The drawing under review shows one solid part. Ordinate dimensions are in mm from its lowest x, y, z. Give positions to 0.01 mm unless a question says otherwise; leave off trailing zeros. Order: outer loops, then holes, each group sorted by start corner. A loop starts at its lowest first (then second) coordinate and runs counter-clockwise, first axis right, second up. Notation, with made-up numbers: (18.25, 25.25) -> (51.25, 25.25) arc R12 cw to (51.25, 42.25) -> close; hole circle Ø5 at (29, 30.5). An arc over 180 degrees is marked (long way). One line per item, written item: value.
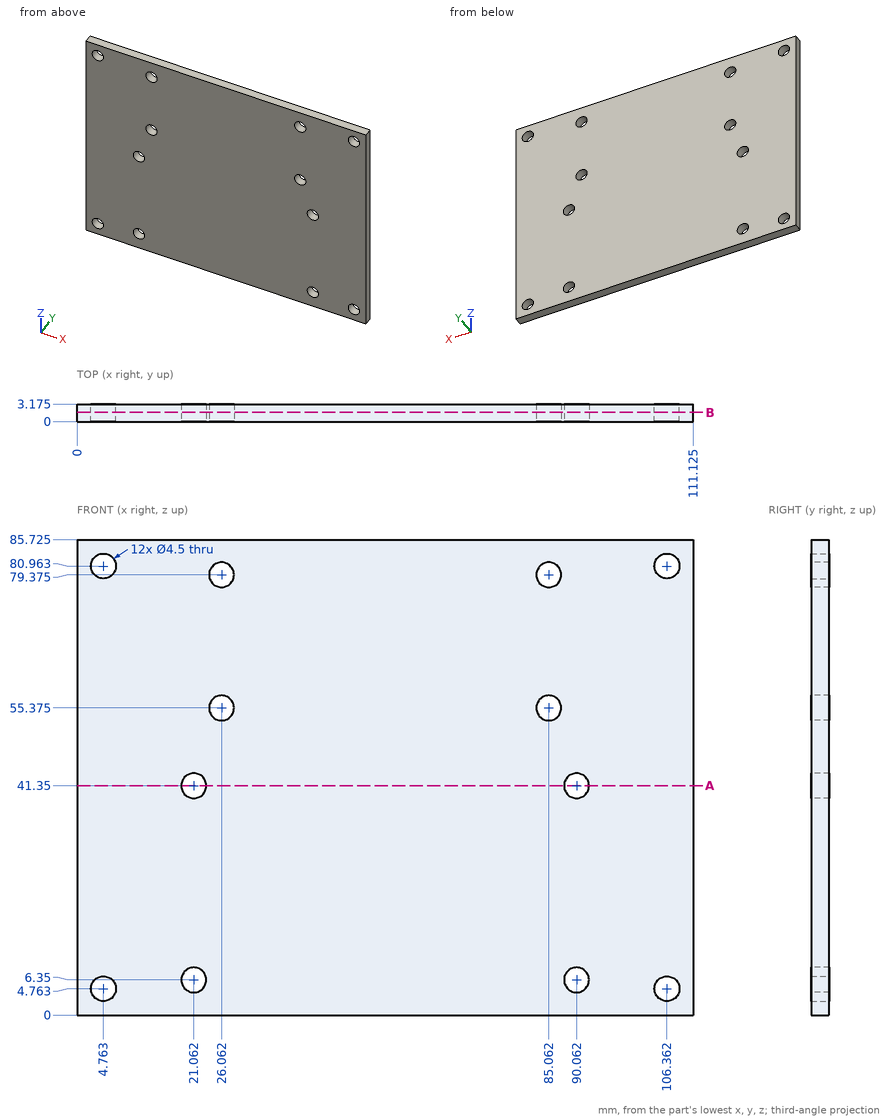
Item 1: Add section A-A on z = 41.35. Give the boundary of the cut face in (x, y) (1 decimal), plus the area to 3 significant figures.
Returned:
outline: (0, 0) -> (18.8, 0) -> (18.8, 3.2) -> (0, 3.2) -> close; (23.3, 0) -> (87.8, 0) -> (87.8, 3.2) -> (23.3, 3.2) -> close; (92.3, 0) -> (111.1, 0) -> (111.1, 3.2) -> (92.3, 3.2) -> close
area: 324 mm²
Item 2: Add section B-B on y = 1.65. Count the separate pieces of the cut face and the enclosed holes in it.
Returned:
separate pieces: 1
enclosed holes: 12
Item 3: To check wall thickness, follow line 1 along X through (y, z) = (0.3, 41.5) (1 decimal); line 2 along Z through (x, y) = (90, 2.8) (1 decimal); line 3 along Z through (x, y) = (25, 2.6) (1 decimal). State the ranges of each line that lie inside material, in increasing order. Write a range as from..to.
Returned:
line 1: 0..18.8, 23.3..87.8, 92.3..111.1
line 2: 0..4.1, 8.6..39.1, 43.6..85.7
line 3: 0..53.4, 57.4..77.4, 81.4..85.7
Item 4: Clearance check with a flat-ended pin moving along its axis: P1, Ø3.5, axis at x = 21.06, z = 6.35, coming from the -Y side. State where the tip first meets the part, or that it passes through.
Returned:
P1: through
